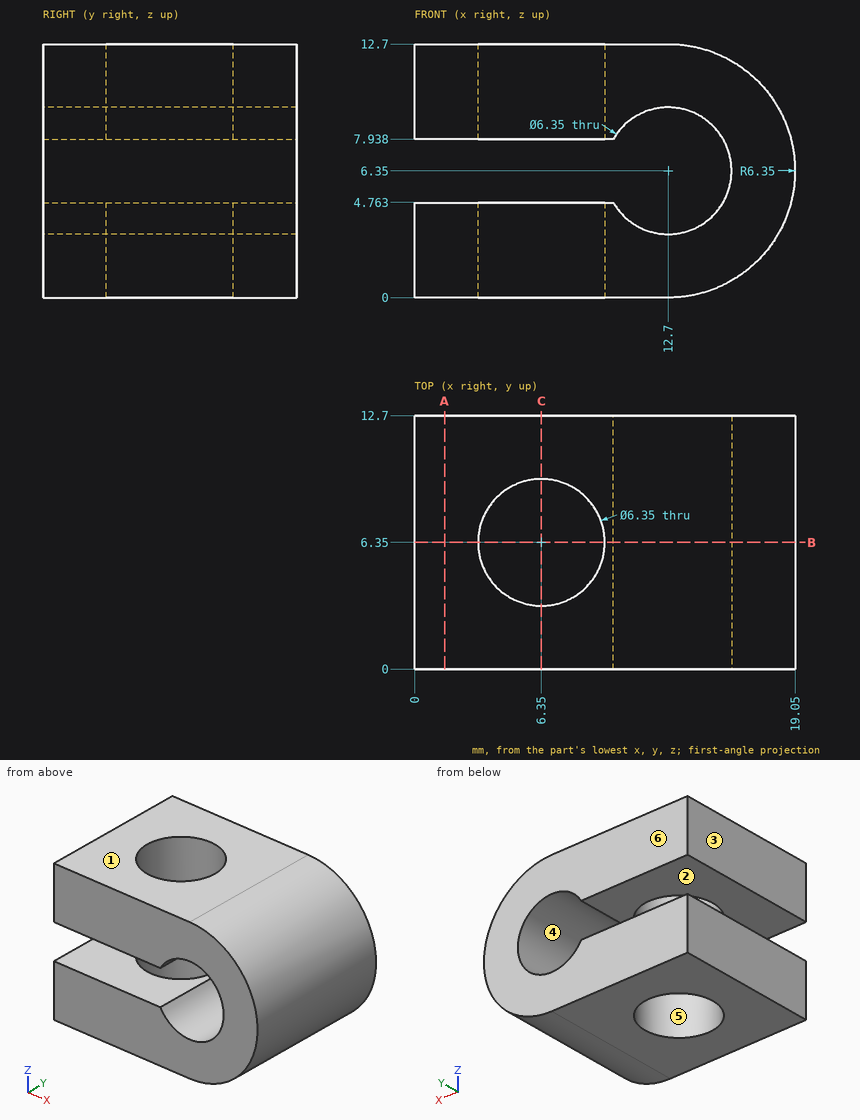
Source: three-view drawing plus pictorial views. Frame: mm from the lowest corner of the part. A direction names the side the tool comes from. Round coordinates to 2 decimals unless told otherwise and drop trailing zeros. Loops run counter-clockwise (first coordinate to the right, second up) from the corner with the lowest first, then second, coordinate; pieces in that order, holes last. Notation, with made-up numbers: M 17.25,53 L 32.25,53 A25 cw 32.25,77 Z; hole C 32.25,84.25 d3. An arc over 180 degrees is marked long. Answer as CSV lines item,"result". Start each with the question number.
(1) First-contact query: pin 1 (3 mm diameter, centred on y = 7, z = 2, fed in from +X) (1 decimal). Flat tip, straight axial feed; report the tip coordinate or a pass-through.
(2) Line query: line 1 (Z direction, x = 1.25, y = 6); line 2 (Y direction, x = 6.35, z = 2.55) (1 decimal); line 3 (Y direction, x = 9, z = 4) (1 decimal). Output: solid intervals per line, ascending. Write a range as [from, to].
(3) Section A-A, the plane x = 1.5. Output: boundary loops of the cut face in (y, z), plus the area to 3 significant figures.
(4) Draft query along X for the marked faces 3, 4, 5 and 6. Return one class per face: released by +X, released by -X, zero draft, split by the parting line, or undercut.
(5) Section B-B, the plane y = 6.35. State how many separate pieces and enclosed holes the cut face has, plus the area to 3 significant figures.
(6) Section C-C, the plane x = 6.35. Output: boundary loops of the cut face in (y, z) (1 decimal).
(7) Reachability of the marked faces 1 and 2 from +Z, -Z, +X, -X, +Y, -Y: full face, straight path, thin tool, end or side. Return the list, or none.
Values found:
1,pin 1,"stops at x = 18.4"
2,line 1,"z = [0, 4.76], [7.94, 12.7]"
2,line 2,"y = [0, 3.2], [9.5, 12.7]"
2,line 3,"y = [0, 4.6], [8.1, 12.7]"
3,outline,"M 0,0 L 12.7,0 L 12.7,4.76 L 0,4.76 Z; M 0,7.94 L 12.7,7.94 L 12.7,12.7 L 0,12.7 Z"
3,area,"121 mm²"
4,face 3,"released by -X"
4,face 4,"undercut"
4,face 5,"undercut"
4,face 6,"zero draft"
5,separate pieces,"3"
5,enclosed holes,"0"
5,area,"102 mm²"
6,outline,"M 0,0 L 3.2,0 L 3.2,4.8 L 0,4.8 Z; M 0,7.9 L 3.2,7.9 L 3.2,12.7 L 0,12.7 Z; M 9.5,0 L 12.7,0 L 12.7,4.8 L 9.5,4.8 Z; M 9.5,7.9 L 12.7,7.9 L 12.7,12.7 L 9.5,12.7 Z"
7,face 1,"+Z, +X, -X, +Y, -Y"
7,face 2,"-X, +Y, -Y"
